```python
from build123d import *

# Parameters (mm, degrees)
EXTRUDE_1_DEPTH     = 10
SKETCH_2_W          = 20
SKETCH_2_H          = 20
SKETCH_2_R          = 1.05
CUT_EXTRUDE_1_DEPTH = 8
SKETCH_2_3_R        = 1.05
CUT_EXTRUDE_2_DEPTH = 235.520787991
SKETCH_3_W          = 30
SKETCH_3_H          = 30
CUT_EXTRUDE_3_DEPTH = 235.520787991


with BuildPart() as part:
    # Sketch 1 → Extrude 1 (new body)
    with BuildSketch(Plane(origin=(0, 0, 0), x_dir=(1, 0, 0), z_dir=(0, 1, 0))):
        Polygon((-150, -120), (20, -120), (20, -180), (80, -180), (80, -120), (150, -120), (150, 120), (-150, 120), align=None)
    extrude(amount=EXTRUDE_1_DEPTH)

    # Sketch 2 → Cut-Extrude 1 (cut)
    with BuildSketch(Plane.XZ):
        with Locations((50, 140)):
            Rectangle(SKETCH_2_W, SKETCH_2_H)
        with Locations(Location((58, 148, 0), (0, 0, 270))):
            Circle(SKETCH_2_R, mode=Mode.SUBTRACT)
        with Locations(Location((42, 148, 0), (0, 0, 270))):
            Circle(SKETCH_2_R, mode=Mode.SUBTRACT)
        with Locations(Location((42, 132, 0), (0, 0, 270))):
            Circle(SKETCH_2_R, mode=Mode.SUBTRACT)
        with Locations(Location((58, 132, 0), (0, 0, 270))):
            Circle(SKETCH_2_R, mode=Mode.SUBTRACT)
    extrude(amount=-CUT_EXTRUDE_1_DEPTH, mode=Mode.SUBTRACT)

    # Sketch 2_3 → Cut-Extrude 2 (cut, through all)
    with BuildSketch(Plane.XZ):
        with Locations(Location((42, 132, 0), (0, 0, 270))):
            Circle(SKETCH_2_3_R)
        with Locations(Location((42, 148, 0), (0, 0, 270))):
            Circle(SKETCH_2_3_R)
        with Locations(Location((58, 132, 0), (0, 0, 270))):
            Circle(SKETCH_2_3_R)
        with Locations(Location((58, 148, 0), (0, 0, 270))):
            Circle(SKETCH_2_3_R)
    extrude(amount=-CUT_EXTRUDE_2_DEPTH, mode=Mode.SUBTRACT)

    # Sketch 3 → Cut-Extrude 3 (cut, through all)
    with BuildSketch(Plane(origin=(0, 10, 0), x_dir=(1, 0, 0), z_dir=(0, 1, 0))):
        with Locations((-85, -60)):
            Rectangle(SKETCH_3_W, SKETCH_3_H)
        with Locations((-85, -10)):
            Rectangle(SKETCH_3_W, SKETCH_3_H)
        with Locations((-85, 40)):
            Rectangle(SKETCH_3_W, SKETCH_3_H)
        with Locations((-85, 90)):
            Rectangle(SKETCH_3_W, SKETCH_3_H)
        with Locations((-15, -60)):
            Rectangle(SKETCH_3_W, SKETCH_3_H)
        with Locations((-15, -10)):
            Rectangle(SKETCH_3_W, SKETCH_3_H)
        with Locations((-15, 40)):
            Rectangle(SKETCH_3_W, SKETCH_3_H)
        with Locations((-15, 90)):
            Rectangle(SKETCH_3_W, SKETCH_3_H)
    extrude(amount=-CUT_EXTRUDE_3_DEPTH, mode=Mode.SUBTRACT)


solid = part.part
```
Input: part model. Units: mm. Frame: model coordinates. A direction names the side the tool comes from. Give positions to 0.01 mm unless a question says otherwise; leave off trailing zeros. Loops run counter-clockwise (first coordinate to the right, second up) from the corner with the lowest first, then second, coordinate; pieces in that order, holes last.
1) Contact query for flat-ended pins moving along their axis: pin 1 (4 mm diameter, centred on y = 3.5, z = 139, fed in from -X); pin 2 (3 mm diameter, centred on x = -19, y = 5.5, fed in from +Z). Output: stop coordinate, or through.
A:
pin 1: stops at x = 20
pin 2: stops at z = 120
2) Section query B-B on x = -92. Return the cut outline in (y, z), and give its area (3 significant figures).
A:
outline: (0, -120) - (10, -120) - (10, -105) - (0, -105) - close; (0, -75) - (10, -75) - (10, -55) - (0, -55) - close; (0, -25) - (10, -25) - (10, -5) - (0, -5) - close; (0, 25) - (10, 25) - (10, 45) - (0, 45) - close; (0, 75) - (10, 75) - (10, 120) - (0, 120) - close
area: 1,200 mm2
3) Line query: L1, parallel to X at y = 6.5, z = -33.5; L2, parallel to X at y = 9.4, z = 132; L3, parallel to Z at x = -10.5, y = 1.25. Output: solid intervals per line, ascending.
A:
L1: x = -150 to -100, -70 to -30, 0 to 150
L2: x = 20 to 40.95, 43.05 to 56.95, 59.05 to 80
L3: z = -120 to -105, -75 to -55, -25 to -5, 25 to 45, 75 to 120
4) Section query D-D on y = 2.25. Count the separate pieces of the cut face and the enclosed holes in it, and give its area (3 significant figures).
A:
separate pieces: 1
enclosed holes: 9
area: 68,000 mm2
5) Reachability of faces 5 (the flat face through (-15, 5, 75)), 6 (the flat face through (-150, 5, -2)), 7 (the flat face through (50, 4, 150)) from +Z, -Z, +X, -X, +Y, -Y: full face, straight path, thin tool, end or side. Return the list, or none.
A:
face 5: +Y, -Y
face 6: +Z, -Z, -X, +Y, -Y
face 7: -Y
6) Mould query, pull axis Z, two halves, no side actions, for faces 1 (the flat face through (80, 5, 150)), 2 (the flat face through (115, 5, 120)), 3 (the flat face through (2, 5, -120)), 4 (the flat face through (50, 8, 140)). Classes: released by +Z, released by -Z, zero draft, split by the parting line, or undercut.
A:
face 1: zero draft
face 2: released by +Z
face 3: released by -Z
face 4: undercut
7) Section query C-C on x = 53. Return the cut outline in (y, z).
A:
outline: (0, -120) - (10, -120) - (10, 180) - (0, 180) - (0, 150) - (8, 150) - (8, 130) - (0, 130) - close
8) Section query A-A on z = -87. Return the cut outline in (x, y), and give its area (3 significant figures).
A:
outline: (-150, 0) - (-100, 0) - (-100, 10) - (-150, 10) - close; (-70, 0) - (-30, 0) - (-30, 10) - (-70, 10) - close; (0, 0) - (150, 0) - (150, 10) - (0, 10) - close
area: 2,400 mm2
